Build history of the part. All positions in model axes, mm. Round coordinates to 2 decimals unless told otherwise and drop trailing zeros. Loops run counter-clockwise (first coordinate to the right, second up) from the corner with the lowest first, then second, coordinate; pieces in that order, holes last. Notation, with made-up numbers: (-33, -8) - (9, -8) arc R14 ccw to (9, 1) - close; hole circle Ø8 at (33, 43.5). An arc over 180 degrees is marked (long way). Answer as CSV lines item,"result". Start each with the question number.
```python
from build123d import *

# Parameters (mm, degrees)
BOSS_EXTRUDE1_DEPTH = 2
SKETCH3_R           = 2
CUT_EXTRUDE1_DEPTH  = 3


with BuildPart() as part:
    # Sketch2 → Boss-Extrude1 (new body)
    with BuildSketch(Plane.XY):
        with BuildLine():
            Line((-10.445641875, -94.122807376), (-12.17064978, -91.748537682))
            ThreePointArc((-12.17064978, -91.748537682), (-9.595543925, -85.642489446), (-4.985379129, -80.882092847))
            ThreePointArc((-4.985379129, -80.882092847), (-4.281750191, -77.918021049), (-1.988595944, -75.912464041))
            ThreePointArc((-1.988595944, -75.912464041), (1.364054662, -72.988805292), (2.410188275, -68.665189788))
            ThreePointArc((2.410188275, -68.665189788), (1.388898621, -64.812163249), (5, -66.5))
            Line((5, -66.5), (5, -80.5))
            ThreePointArc((5, -80.5), (3.535533906, -84.035533906), (0, -85.5))
            ThreePointArc((0, -85.5), (-6.77244862, -87.934189562), (-10.445641875, -94.122807376))
        make_face()
    extrude(amount=-BOSS_EXTRUDE1_DEPTH)

    # Sketch3 → Cut-Extrude1 (cut, through all)
    with BuildSketch(Plane.XY):
        with Locations((0, -80.5)):
            Circle(SKETCH3_R)
    extrude(amount=-CUT_EXTRUDE1_DEPTH, mode=Mode.SUBTRACT)


solid = part.part
```
Q1. Band-saw the part on D-D, the plane x = 2.8. List the corners of the cut face in (y, z), then the cut area to 3 significant figures.
Q2. Two-plate mould, pull along Y, no slides. Class faces 1 (the cylindrical face through (-0.26, -78.517, -0.986)), 2 (the cylindrical face through (3.57, -84, -0.99)), 3 (the flat face through (-2, -79, 0)): released by +Y, released by -Y, zero draft, split by the parting line, or undercut.
Q3. Band-saw the part on B-B, the plane z = -1.7. List the corners of the cut face in (x, y), then the cut area to 3 significant figures.
Q4. Band-saw the part on C-C, the plane y = -76.5. List the corners of the cut face in (x, z).
Q5. Band-saw the part on A-A, the plane y = -79.5. List the corners of the cut face in (x, z), then the cut area to 3 significant figures.
Q6. Wall check: probe 1 along Y at (x, z) = (1.25, -1.7); probe 2 along Y at (x, z) = (1.5, -0.25); probe 3 along X at (y, z) = (-81.75, -1.4). Give the ranges that are in metal, low to high. Write a range as [from, to].
Q7. Pin check, flat tip, straight feed: pin 1 Ø2 at (x, y) = (-2.5, -87) entering from -Z. Stop position of the tip, or through.
Reported:
1,outline,"(-84.64, -2) - (-64.3, -2) - (-64.3, 0) - (-84.64, 0) - close"
1,area,"40.7 mm2"
2,face 1,"undercut"
2,face 2,"released by -Y"
2,face 3,"zero draft"
3,outline,"(-12.17, -91.75) - (-10.45, -94.12) arc R10.64 cw to (0, -85.5) arc R5 ccw to (5, -80.5) - (5, -66.5) arc R2.2 ccw (long way) to (2.41, -68.67) arc R7.33 cw to (-1.99, -75.91) arc R5 ccw to (-4.99, -80.88) arc R18 ccw to start; hole circle Ø4 at (0, -80.5)"
3,area,"157 mm2"
4,outline,"(-3, -2) - (5, -2) - (5, 0) - (-3, 0) - close"
5,outline,"(-4.9, -2) - (-1.73, -2) - (-1.73, 0) - (-4.9, 0) - close; (1.73, -2) - (5, -2) - (5, 0) - (1.73, 0) - close"
5,area,"12.9 mm2"
6,probe 1,"y = [-85.34, -82.06], [-78.94, -73.17], [-68.06, -64.94]"
6,probe 2,"y = [-85.27, -81.82], [-79.18, -72.76], [-68.27, -64.73]"
6,probe 3,"x = [-6.11, -1.56], [1.56, 4.84]"
7,pin 1,"passes through"
